Input: part model. Units: mm. Frame: model coordinates. A direction names the side the tool comes from. Round coordinates to 2 decimals unless told otherwise and drop trailing zeros. Loops run counter-clockwise (first coordinate to the right, second up) from the corner with the lowest first, then second, coordinate; pieces in that order, holes last. Notation, with made-up numbers: (34, -24.5) -> (61, -24.5) arc R17 cw to (61, -5.5) -> close; hole circle Ø2 at (40, -18.5). An arc over 180 degrees is marked (long way). Answer in a Markdown table with one row per item. Add a question column.
Q1. Pin query (flat end, axial travel): pin 1 (0.9 mm diameter, centred on y = 2, z = -21, fed in from -X); pin 2 (0.9 mm diameter, centred on y = 1, z = 12.5, fed in from -X); pin 3 (0.9 mm diameter, centred on y = 1, z = -20, fed in from +X). Return the tip coordinate at first contact, or that it passes through.
Q2. Ray query, L1, parallel to X at y = 0.85, z = -19.5; L2, parallel to Z at x = 0, y = 1.2; L3, parallel to X at y = 1.35, z = -6. Return the intervals inside material, ascending. Write a range as from..to.
Q3. Section C-C, the plane z = -19. Output: boundary loops of the cut face in (x, y), and give its area (3 significant figures).
Q4. Section A-A, the plane x = 0. Output: boundary loops of the cut face in (y, z), and give its area (3 significant figures).
Q5. Section B-B, the plane z = 12. Output: boundary loops of the cut face in (x, y).
Q6. Reachability of faces 1 (the face through (17.5, 1, 8)), 2 (the face through (-17.5, 1, 8)), 3 (the face through (-20, 2, -17.5)) from +Z, -Z, +X, -X, +Y, -Y: full face, straight path, thin tool, end or side. Return the list, or none.
Q7. Section D-D, the plane x = -11. Output: boundary loops of the cut face in (y, z), and give its area (3 significant figures).
Q8. Mould query, pull axis X, two halves, no side actions, for faces 4 (the face through (0, 1, 17.5)), 5 (the face through (4.57, 1.521, -7.167)), 6 (the face through (12.5, 2, -20)), 7 (the face through (-0.325, 1.521, 13.464)). Classes: pulls with the +X half, pulls with the -X half, needs draft (parallel to the pull), parting line crosses it, or undercut.
```python
from build123d import *

# Parameters (mm, degrees)
ESQUISSE1_W                = 35
ESQUISSE1_H                = 35
BOSS_EXTRU_1_DEPTH         = 3
ESQUISSE2_W                = 5
ESQUISSE2_H                = 5
BOSS_EXTRU_2_DEPTH         = 3
R_P_TITION_LIN_AIRE1_COUNT = 3
R_P_TITION_LIN_AIRE1_PITCH = 10
ESQUISSE3_R                = 8.5
ESQUISSE3_R_2              = 1.5
ENL_V_MAT_EXTRU_1_DEPTH    = 5
ESQUISSE4_W                = 10
ESQUISSE4_H                = 16.5
BOSS_EXTRU_3_DEPTH         = 3


with BuildPart() as part:
    # Esquisse1 → Boss.-Extru.1 (new body)
    with BuildSketch(Plane(origin=(0, 0, 0), x_dir=(1, 0, 0), z_dir=(0, 1, 0))):
        Rectangle(ESQUISSE1_W, ESQUISSE1_H)
    extrude(amount=BOSS_EXTRU_1_DEPTH)

    # Esquisse2 → Boss.-Extru.2 (add)
    with BuildSketch(Plane(origin=(0, 3, 0), x_dir=(1, 0, 0), z_dir=(0, 1, 0))):
        with Locations((-10, 20)):
            Rectangle(ESQUISSE2_W, ESQUISSE2_H)
    boss_extru_2 = extrude(amount=-BOSS_EXTRU_2_DEPTH)

    # Répétition linéaire1: Boss.-Extru.2 ×3
    with Locations(*[(i * R_P_TITION_LIN_AIRE1_PITCH, 0, 0) for i in range(1, R_P_TITION_LIN_AIRE1_COUNT)]):
        add(boss_extru_2)

    # Esquisse3 → Enlèv. mat.-Extru.1 (cut)
    with BuildSketch(Plane(origin=(0, 3, 0), x_dir=(1, 0, 0), z_dir=(0, 1, 0))):
        Circle(ESQUISSE3_R)
        with Locations((0, -12)):
            Circle(ESQUISSE3_R_2)
        with Locations((-10.392304845, 6)):
            Circle(ESQUISSE3_R_2)
        with Locations((10.392304845, 6)):
            Circle(ESQUISSE3_R_2)
    extrude(amount=-ENL_V_MAT_EXTRU_1_DEPTH, mode=Mode.SUBTRACT)

    # Esquisse4 → Boss.-Extru.3 (add)
    with BuildSketch(Plane(origin=(0, 3, 0), x_dir=(1, 0, 0), z_dir=(0, 1, 0))):
        with Locations((-22.5, 9.25)):
            Rectangle(ESQUISSE4_W, ESQUISSE4_H)
    boss_extru_3 = extrude(amount=-BOSS_EXTRU_3_DEPTH)

    # Symétrie1: Boss.-Extru.3 across plane
    add(boss_extru_3.mirror(Plane(origin=(0, 0, 0), x_dir=(0, 0, 1), z_dir=(1, 0, 0))))


solid = part.part
```
Answer block:
| question | item | result |
|---|---|---|
| 1 | pin 1 | x = -12.5 |
| 1 | pin 2 | x = -17.5 |
| 1 | pin 3 | x = 12.5 |
| 2 | L1 | -12.5..-7.5, -2.5..2.5, 7.5..12.5 |
| 2 | L2 | -22.5..-8.5, 8.5..10.5, 13.5..17.5 |
| 2 | L3 | -27.5..-11.89, -8.89..-6.02, 6.02..8.89, 11.89..27.5 |
| 3 | outline | (-12.5, 0) -> (-7.5, 0) -> (-7.5, 3) -> (-12.5, 3) -> close; (-2.5, 0) -> (2.5, 0) -> (2.5, 3) -> (-2.5, 3) -> close; (7.5, 0) -> (12.5, 0) -> (12.5, 3) -> (7.5, 3) -> close |
| 3 | area | 45.0 mm^2 |
| 4 | outline | (0, -22.5) -> (3, -22.5) -> (3, -8.5) -> (0, -8.5) -> close; (0, 8.5) -> (3, 8.5) -> (3, 10.5) -> (0, 10.5) -> close; (0, 13.5) -> (3, 13.5) -> (3, 17.5) -> (0, 17.5) -> close |
| 4 | area | 60.0 mm^2 |
| 5 | outline | (-17.5, 0) -> (-1.5, 0) -> (-1.5, 3) -> (-17.5, 3) -> close; (1.5, 0) -> (17.5, 0) -> (17.5, 3) -> (1.5, 3) -> close |
| 6 | face 1 | +Z, +X, +Y, -Y |
| 6 | face 2 | +Z, -X, +Y, -Y |
| 6 | face 3 | -Z, -X, +Y, -Y |
| 7 | outline | (0, -22.5) -> (3, -22.5) -> (3, -7.37) -> (0, -7.37) -> close; (0, -4.63) -> (3, -4.63) -> (3, 17.5) -> (0, 17.5) -> close |
| 7 | area | 112 mm^2 |
| 8 | face 4 | needs draft |
| 8 | face 5 | undercut |
| 8 | face 6 | pulls with the +X half |
| 8 | face 7 | undercut |
